Here's how the part is built. I have some questions about the finished solid (model axes, mm). A direction names the side the tool comes from. Round coordinates to 2 decimals unless told otherwise and drop trailing zeros. Order: outer loops, then holes, each group sorted by start corner. A loop starts at its lowest first (then second) coordinate and runs counter-clockwise, first axis right, second up. Notation, with made-up numbers: (-31, 36.25) -> (-23, 36.25) arc R20 ccw to (-23, 68.25) -> close; hole circle Ø7 at (69.5, 81.5). An arc over 180 degrees is marked (long way). Answer in a Markdown table with one row per item.
```python
from build123d import *

# Parameters (mm, degrees)
F1_DEPTH = 5
F2_W     = 6.4714387385
F2_H     = 11.8567999452
F2_W_2   = 12.5
F2_H_2   = 9.7434073687
F3_DEPTH = 5


# Not quite as in the source:
# - ends of sketch curves that miss each other by under 0.0002 mm in the source are joined
# - a feature names something its author has since deleted; it is built from what else it names


with BuildPart() as f1:
    # F0 (on Top) → F1 (new body)
    with BuildSketch(Plane.XY):
        with BuildLine():
            Line((0, 29.2999204248), (0, 0))
            Line((0, 0), (34.4714387385, 0))
            Line((34.4714387385, 0), (34.4714387385, 16.3473710418))
            ThreePointArc((34.4714387385, 16.3473710418), (32.5790927131, 15.1300794804), (32.2559916738, 17.3568210333))
            ThreePointArc((32.2559916738, 17.3568210333), (15.182844974, 14.8438668457), (5.7578901922, 29.2999210911))
            ThreePointArc((5.7578901922, 29.2999210911), (2.8789043427, 26.4210160822), (0, 29.2999204248))
        make_face()
        with BuildLine():
            ThreePointArc((5.7577396052, 29.3198639813), (2.8689325046, 32.1788074974), (0, 29.2999204248))
            ThreePointArc((0, 29.2999204248), (2.8789043427, 26.4210160822), (5.7578086853, 29.2999204248))
            ThreePointArc((5.7578086853, 29.2999204248), (5.7578117914, 29.3098925127), (5.7577396052, 29.3198639813))
        make_face()
        with BuildLine():
            ThreePointArc((32.2559916738, 17.3568210333), (32.5790927131, 15.1300794804), (34.4714387385, 16.3473710418))
            ThreePointArc((34.4714387385, 16.3473710418), (33.6883902233, 17.5646626032), (32.2559916738, 17.3568210333))
        make_face()
    extrude(amount=F1_DEPTH)

    # F2 (on face) → F3 (join)
    with BuildSketch(Plane.XY.offset(5)):
        with BuildLine():
            Line((28, 0), (34.4714387385, 0))
            Line((34.4714387385, 0), (34.4714387385, 16.3473710418))
            ThreePointArc((34.4714387385, 16.3473710418), (33.6883902233, 17.5646626032), (32.2559916738, 17.3568210333))
            ThreePointArc((32.2559916738, 17.3568210333), (15.182844974, 14.8438668457), (5.7578901922, 29.2999210911))
            ThreePointArc((5.7578901922, 29.2999210911), (5.757811792, 29.3098923335), (5.7577396052, 29.3198639813))
            ThreePointArc((5.7577396052, 29.3198639813), (2.8689325046, 32.1788074974), (0, 29.2999204248))
            Line((0, 29.2999204248), (0, 25.3991372883))
            Line((0, 25.3991372883), (0, 0))
            Line((0, 0), (12.5, 0))
            Line((12.5, 0), (28, 0))
        make_face()
        with Locations((31.2357193692, -5.9283999726)):
            Rectangle(F2_W, F2_H)
        with Locations((6.25, -5.9283999726)):
            Rectangle(F2_W_2, F2_H)
        with Locations((6.25, -16.7285036296)):
            Rectangle(F2_W_2, F2_H_2)
        with Locations((6.25, -5.9283999726)):
            Rectangle(F2_W_2, F2_H)
    extrude(amount=-F3_DEPTH)


solid = f1.part
```
1. Please list where these lines run through material, in increasing order: line 1 along X through (y, z) = (-10.5, 4.15); line 2 along X through (y, z) = (-15.5, 1.2); line 3 along X through (y, z) = (16.5, 4.25).
Numbers:
| item | result |
|---|---|
| line 1 | x = 0 to 12.5, 28 to 34.47 |
| line 2 | x = 0 to 12.5 |
| line 3 | x = 0 to 12.33, 31.18 to 34.46 |
2. Suppose I cut it at A-A on y = -5. Write out the boundary of the cut face in (x, z), then the cut area to 3 significant figures.
Numbers:
| item | result |
|---|---|
| outline | (0, 0) -> (12.5, 0) -> (12.5, 5) -> (0, 5) -> close; (28, 0) -> (34.47, 0) -> (34.47, 5) -> (28, 5) -> close |
| area | 94.9 mm2 |
3. For pin 1 Ø2 at (y, z) = (-15, 2.5) entering from +X, with a flat end and sliding along its axis, tell me the tip position at first contact or that it passes through.
Numbers:
| item | result |
|---|---|
| pin 1 | stops at x = 12.5 |
4. For faces 1 (the face through (28, -6, 3)), 2 (the face through (31, -11.857, 3)), 3 (the face through (13, 6, 0)), which set-ups out of +Z, -Z, +X, -X, +Y, -Y let a thin tool reach every point of the face, with its end or its side?
Numbers:
| item | result |
|---|---|
| face 1 | +Z, -Z, -Y |
| face 2 | +Z, -Z, +X, -Y |
| face 3 | -Z, +X, -X, +Y, -Y |
5. Suppose I cut it at C-C on x = 31.5. Write out the boundary of the cut face in (y, z).
Numbers:
| item | result |
|---|---|
| outline | (-11.86, 0) -> (16.74, 0) -> (16.74, 5) -> (-11.86, 5) -> close |
6. Suppose I cut it at D-D on y = -15.5. Write out the boundary of the cut face in (x, z).
Numbers:
| item | result |
|---|---|
| outline | (0, 0) -> (12.5, 0) -> (12.5, 5) -> (0, 5) -> close |
